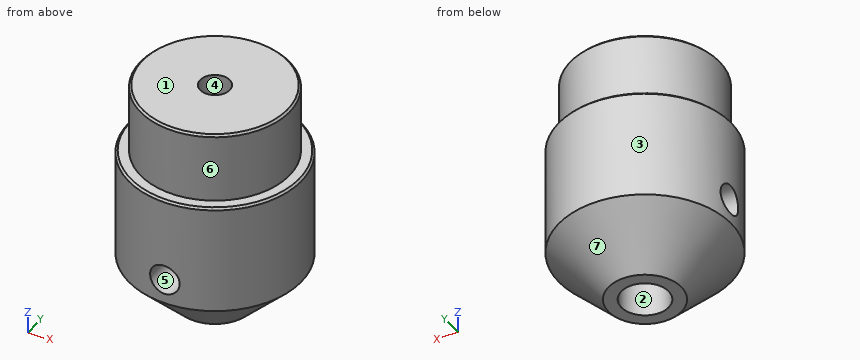
```python
from build123d import *

# Parameters (mm, degrees)
SKETCH1_R                    = 10.9982
BOSS_EXTRUDE1_DEPTH          = 20.32
SKETCH2_R                    = 9.4996
BOSS_EXTRUDE2_DEPTH          = 8.89
B_0_238_DIAMETER_HOLE1_D     = 6.0452
B_0_238_DIAMETER_HOLE1_DEPTH = 19.05
B_0_238_DIAMETER_HOLE1_TIP   = 1.816161307
BOSS_EXTRUDE5_START          = -9.484662807
BOSS_EXTRUDE5_OUTLINE_R      = 1.89865
BOSS_EXTRUDE5_DEPTH          = 9.484662807
SKETCH11_R                   = 1.89865
CUT_EXTRUDE1_DEPTH           = 34.092973672
SKETCH12_R                   = 1.89865
CUT_EXTRUDE2_DEPTH           = 34.092973739
CHAMFER1_SIZE                = 6.35
CHAMFER2_SIZE                = 0.254
CHAMFER3_SIZE                = 0.254


# Read off the part's stored shape, not the designer's step: Boss-Extrude5
with BuildPart() as part:
    # Sketch1 → Boss-Extrude1 (new body)
    with BuildSketch(Plane.XY):
        Circle(SKETCH1_R)
    extrude(amount=BOSS_EXTRUDE1_DEPTH)

    # Sketch2 → Boss-Extrude2 (add)
    with BuildSketch(Plane.XY.offset(20.32)):
        Circle(SKETCH2_R)
    extrude(amount=BOSS_EXTRUDE2_DEPTH)

    # B (0.238) Diameter Hole1
    with Locations(Plane(origin=(0, 0, 0), x_dir=(-1, 0, 0), z_dir=(0, 0, -1))):
        with Locations((0, 0)):
            Hole(B_0_238_DIAMETER_HOLE1_D / 2, depth=B_0_238_DIAMETER_HOLE1_DEPTH)
            with Locations((0, 0, -(B_0_238_DIAMETER_HOLE1_DEPTH + B_0_238_DIAMETER_HOLE1_TIP / 2))):  # 118° drill point
                Cone(0, B_0_238_DIAMETER_HOLE1_D / 2, B_0_238_DIAMETER_HOLE1_TIP, mode=Mode.SUBTRACT)

    # Boss-Extrude5 outline → Boss-Extrude5 (cut)
    with BuildSketch(Plane.XY.offset(29.21).offset(BOSS_EXTRUDE5_START)):
        Circle(BOSS_EXTRUDE5_OUTLINE_R)
    extrude(amount=BOSS_EXTRUDE5_DEPTH, mode=Mode.SUBTRACT)

    # Sketch11 → Cut-Extrude1 (cut, through all)
    with BuildSketch(Plane(origin=(0, 0, 0), x_dir=(1, 0, 0), z_dir=(0, 1, 0))):
        with Locations(Location((0, -9.525, 0), (0, 0, 270))):
            Circle(SKETCH11_R)
    extrude(amount=-CUT_EXTRUDE1_DEPTH, mode=Mode.SUBTRACT)

    # Sketch12 → Cut-Extrude2 (cut, through all)
    with BuildSketch(Plane(origin=(0, 0, 0), x_dir=(0, 0, -1), z_dir=(1, 0, 0))):
        with Locations((-9.525, 0)):
            Circle(SKETCH12_R)
    extrude(amount=-CUT_EXTRUDE2_DEPTH, mode=Mode.SUBTRACT)

    # Chamfer1
    chamfer1_edges = [part.edges().sort_by_distance(p)[0] for p in [
        (-10.9982, 0, 0),
    ]]
    chamfer(chamfer1_edges, length=CHAMFER1_SIZE)

    # Chamfer2
    chamfer2_edges = [part.edges().sort_by_distance(p)[0] for p in [
        (-10.9982, 0, 20.32),
    ]]
    chamfer(chamfer2_edges, length=CHAMFER2_SIZE)

    # Chamfer3
    chamfer3_edges = [part.edges().sort_by_distance(p)[0] for p in [
        (-9.4996, 0, 29.21),
    ]]
    chamfer(chamfer3_edges, length=CHAMFER3_SIZE)


solid = part.part
```
The listing builds one solid part. Answer for the finished solid, in the listing's coordinates (mm). Face numbers are marked on the shaded views. A direction names the side the tool comes from. Give positions to 0.01 mm unless a question says otherwise; leave off trailing zeros. Order: outer loops, then holes, each group sorted by start corner. A loop starts at its lowest first (then second) coordinate and runs counter-clockwise, first axis right, second up. Notation, with made-up numbers: (69.5, -5) - (92.5, -5) arc R14 cw to (92.5, 20) - close; hole circle Ø8 at (22, -21). An arc over 180 degrees is marked (long way). Answer in a Markdown table with one row per item. Add a question column.
Q1. For a pull along X with two mould halves and no side action, classify the marked faces 1, 2, 3 and 4 as released by +X, released by -X, zero draft, split by the parting line, or undercut.
Q2. The part is cut by section A-A (x = 0). Determine the outline of the cut face in (y, z), then the cut area to 3 significant figures.
Q3. Find the intervals of material crossed by line 1 along Y through (x, z) = (0, 21.5); line 2 along Y through (x, z) = (0, 14); line 3 along X through (y, z) = (0, 8), in increasing order. Write a range as [from, to].
Q4. The part is cut by section C-C (z = 26). Determine the outline of the cut face in (x, y).
Q5. Given P1, Ø3, axis at y = 7.5, z = 20, coming from the -X side; P2, Ø3, axis at x = 7.5, z = 12.5, coming from the +Y side; P3, Ø3, axis at x = 8, y = 3.5, coming from the -Z side, each flat-ended and moving along its own axis, determine where each tip first touches the part or whether it passes through.
Q6. Which of the six approach directions +Z, -Z, +X, -X, +Y, -Y give full straight-line access (tool end or side, diameter ignored) to the marked faces 5, 6 and 7?
Q7. The part is cut by section D-D (z = 14.75). Determine the outline of the cut face in (x, y).
Determined:
| question | item | result |
|---|---|---|
| 1 | face 1 | zero draft |
| 1 | face 2 | undercut |
| 1 | face 3 | split by the parting line |
| 1 | face 4 | undercut |
| 2 | outline | (-11, 6.35) - (-4.65, 0) - (-3.02, 0) - (-3.02, 7.63) - (-11, 7.63) - close; (-11, 11.42) - (-3.02, 11.42) - (-3.02, 19.05) - (-1.9, 19.73) - (-1.9, 29.21) - (-9.25, 29.21) - (-9.5, 28.96) - (-9.5, 20.32) - (-10.74, 20.32) - (-11, 20.07) - close; (1.9, 19.73) - (3.02, 19.05) - (3.02, 0) - (4.65, 0) - (11, 6.35) - (11, 20.07) - (10.74, 20.32) - (9.5, 20.32) - (9.5, 28.96) - (9.25, 29.21) - (1.9, 29.21) - close |
| 2 | area | 391 mm² |
| 3 | line 1 | y = [-9.5, -1.9], [1.9, 9.5] |
| 3 | line 2 | y = [-11, -3.02], [3.02, 11] |
| 3 | line 3 | x = [3.02, 11] |
| 4 | outline | circle Ø19 at (0, 0); hole circle Ø3.8 at (0, 0) |
| 5 | P1 | stops at x = -9.22 |
| 5 | P2 | stops at y = 9.22 |
| 5 | P3 | stops at z = 2.58 |
| 6 | face 5 | -Y |
| 6 | face 6 | +Z |
| 6 | face 7 | -Z |
| 7 | outline | circle Ø22 at (0, 0); hole circle Ø6.05 at (0, 0) |
